Verification items for the finished model (mm, model axes). Face numbers are marked on the shaded views. A direction names the side the tool comes from. Round coordinates to 2 decimals unless told otherwise and drop trailing zeros. Loops run counter-clockwise (first coordinate to the right, second up) from the corner with the lowest first, then second, coordinate; pieces in that order, holes last. Notation, with made-up numbers: (-36, -15) - (-1, -15) arc R11 cw to (-1, 6) - close; hole circle Ø5 at (-40, 80). An arc over 180 degrees is marked (long way). Use CSV: the item, a comma, the result in double quotes.
```python
from build123d import *

# Parameters (mm, degrees)
SKETCH_1_R               = 1.6
EXTRUDE_1_DEPTH          = 3
SKETCH_4_R               = 14
EXTRUDE_2_DEPTH          = 7
CUT_EXTRUDE_1_DEPTH      = 54.460265618
CUT_EXTRUDE_1_DEPTH_BACK = 54.460265618
SKETCH_2_R               = 7.5
SKETCH_3_R               = 1.6
CUT_EXTRUDE_2_DEPTH      = 54.460265618


with BuildPart() as part:
    # ｽｹｯﾁ1 → ﾎﾞｽ - 押し出し1 (new body)
    with BuildSketch(Plane(origin=(0, 0, 0), x_dir=(1, 0, 0), z_dir=(0, 1, 0))):
        with BuildLine():
            Line((5, 40), (5, 27.549954628))
            ThreePointArc((5, 27.549954628), (28, 0), (5, -27.549954628))
            Line((5, -27.549954628), (5, -40))
            ThreePointArc((5, -40), (0, -45), (-5, -40))
            Line((-5, -40), (-5, -27.549954628))
            ThreePointArc((-5, -27.549954628), (-28, 0), (-5, 27.549954628))
            Line((-5, 27.549954628), (-5, 40))
            ThreePointArc((-5, 40), (0, 45), (5, 40))
        make_face()
        with Locations(Location((0, 40, 0), (0, 0, 270))):
            Circle(SKETCH_1_R, mode=Mode.SUBTRACT)
        with Locations(Location((0, -40, 0), (0, 0, 270))):
            Circle(SKETCH_1_R, mode=Mode.SUBTRACT)
    extrude(amount=EXTRUDE_1_DEPTH)

    # ｽｹｯﾁ4 → ﾎﾞｽ - 押し出し2 (add)
    with BuildSketch(Plane(origin=(0, 3, 0), x_dir=(1, 0, 0), z_dir=(0, 1, 0))):
        with Locations(Location((7, 0, 0), (0, 0, 270))):
            Circle(SKETCH_4_R)
    extrude(amount=EXTRUDE_2_DEPTH)

    # ｽｹｯﾁ2 → ｶｯﾄ - 押し出し1 (cut, two sides: drawn at the far end of the back side and taken through both)
    with BuildSketch(Plane(origin=(0, 3, 0), x_dir=(1, 0, 0), z_dir=(0, 1, 0)).offset(-CUT_EXTRUDE_1_DEPTH_BACK)):
        with Locations(Location((7, 0, 0), (0, 0, 270))):
            Circle(SKETCH_2_R)
    extrude(amount=CUT_EXTRUDE_1_DEPTH + CUT_EXTRUDE_1_DEPTH_BACK, mode=Mode.SUBTRACT)

    # ｽｹｯﾁ3 → ｶｯﾄ - 押し出し2 (cut, through all)
    with BuildSketch(Plane(origin=(0, 3, 0), x_dir=(1, 0, 0), z_dir=(0, 1, 0))):
        with Locations(Location((-23, 0, 0), (0, 0, 270))):
            Circle(SKETCH_3_R)
        with Locations(Location((11.5, 19.918584287, 0), (0, 0, 270))):
            Circle(SKETCH_3_R)
        with Locations(Location((11.5, -19.918584287, 0), (0, 0, 270))):
            Circle(SKETCH_3_R)
    extrude(amount=-CUT_EXTRUDE_2_DEPTH, mode=Mode.SUBTRACT)


solid = part.part
```
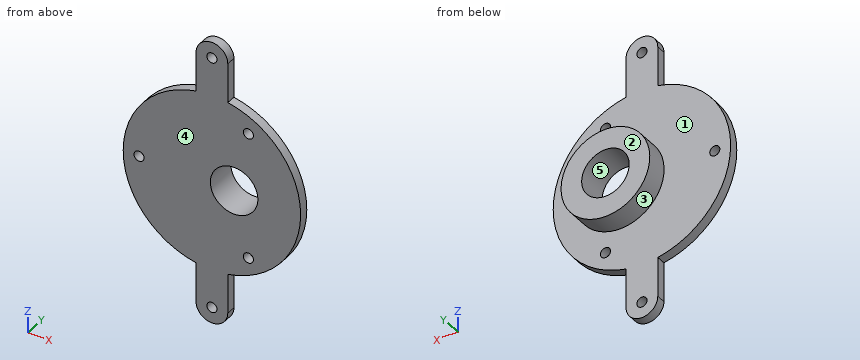
1) Cross-section at A-A, the plane z = 0. Record the cut outline in (x, y), then the cut area to 3 significant figures.
Returned:
outline,"(-28, 0) - (-24.6, 0) - (-24.6, 3) - (-28, 3) - close; (-21.4, 0) - (-0.5, 0) - (-0.5, 10) - (-7, 10) - (-7, 3) - (-21.4, 3) - close; (14.5, 0) - (28, 0) - (28, 3) - (21, 3) - (21, 10) - (14.5, 10) - close"
area,"204 mm²"
2) Cross-section at D-D, the plane y = 5. Record the cut outline in (x, z), then the cut area to 3 significant figures.
Returned:
outline,"circle Ø28 at (7, 0); hole circle Ø15 at (7, 0)"
area,"439 mm²"
3) Thickness scan on probe 1 along X at (y, z) = (0.9, 40); probe 2 along X at (y, z) = (0.95, 0); probe 3 along Z at (x, y) = (12, 1). Record the ranges inside material, lowest first. Write a range as [from, to].
Returned:
probe 1,"x = [-5, -1.6], [1.6, 5]"
probe 2,"x = [-28, -24.6], [-21.4, -0.5], [14.5, 28]"
probe 3,"z = [-25.3, -21.44], [-18.4, -5.59], [5.59, 18.4], [21.44, 25.3]"
4) Mould release check, pull along X, two halves, no side actions. Record for the marked faces 3, 4 and 5: +X half, -X half, draft (parallel to the pull), parting line (faces both ways), or undercut.
Returned:
face 3,"parting line"
face 4,"draft"
face 5,"undercut"
5) Cross-section at C-C, the plane x = -23. Record the cut outline in (y, z).
Returned:
outline,"(0, -15.97) - (3, -15.97) - (3, -1.6) - (0, -1.6) - close; (0, 1.6) - (3, 1.6) - (3, 15.97) - (0, 15.97) - close"
6) Access from +Z, -Z, +X, -X, +Y, -Y to the whole of each face (thin tool, end or side, straight path). Record for the marked faces 1 and 2.
Returned:
face 1,"+Y"
face 2,"+Z, -Z, +X, -X, +Y"
7) Gauge pin test, flat ends, axial feed: pin 1 Ø1.5 at (y, z) = (2, -34.5) entering from -X; pin 2 Ø3 at (y, z) = (7, 11.5) entering from -X; pin 3 Ø3.5 at (y, z) = (1.5, 32) entering from +X. Record the tip position at first contact, or that the pin passes through.
Returned:
pin 1,"stops at x = -5"
pin 2,"stops at x = -2.8"
pin 3,"stops at x = 5"
8) Cross-section at B-B, the plane y = 1.25. Record the cut outline in (x, z).
Returned:
outline,"(-5, -40) arc R5 ccw to (5, -40) - (5, -27.55) arc R28 ccw to (5, 27.55) - (5, 40) arc R5 ccw to (-5, 40) - (-5, 27.55) arc R28 ccw to (-5, -27.55) - close; hole circle Ø3.2 at (-23, 0); hole circle Ø3.2 at (0, -40); hole circle Ø3.2 at (0, 40); hole circle Ø15 at (7, 0); hole circle Ø3.2 at (11.5, -19.92); hole circle Ø3.2 at (11.5, 19.92)"
